The listing builds one solid part. Answer for the finished solid, in the listing's coordinates (mm). Face numbers are marked on the shaded views. A direction names the side the tool comes from. Give positions to 0.01 mm unless a question says otherwise; leave off trailing zeros. Write each loop counter-clockwise with the first axis right and the second up, starting at its lowest first coordinate (ties: lowest second). Pieces come first, ordered by that corner, then holes. Notation, with made-up numbers: (31, 26) - (74, 26) arc R20 ccw to (74, 32) - close; hole circle Ø4 at (51.5, -29.5). An arc over 180 degrees is marked (long way). Use a Markdown table: item, result. Add a question column.
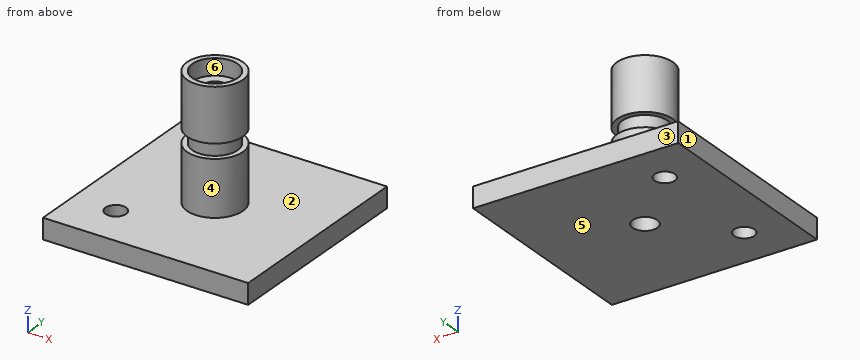
Autodesk Inventor part; units mm, degrees
ref_plane "Plano de trabajo1" through (0, 0, 13.5) normal (0, 0, -1) x (-1, 0, 0)
ref_plane "YZ Plane" through (0, 0, 0) normal (1, 0, 0) x (0, 1, 0)
ref_plane "XZ Plane" through (0, 0, 0) normal (0, 1, 0) x (-1, 0, 0)
sketch "Boceto1" plane through (0, 0, 0) normal (0, 0, 1) x (1, 0, 0)
  circle A0 centre (0, 0) radius 6.8
  dimension "d0" = 13.6
extrude "Extrusión1" add sketch "Boceto1" along normal blind 30
ref_plane "Plano de trabajo1" through (0, 0, 13.5) normal (0, 0, -1) x (-1, 0, 0)
sketch "Boceto2" plane through (0, 0, 13.5) normal (0, 0, -1) x (-1, 0, 0)
  circle A0 centre (0, 0) radius 5.5
  circle A1 centre (0, 0) radius 7
  dimension "d4" = 11
  dimension "d5" = 14
extrude "Extrusión2" cut sketch "Boceto2" against normal blind 3.5
sketch "Boceto3" plane through (0, 0, 0) normal (0, 0, -1) x (-1, 0, 0)
  line L0 (-25, 25) -> (25, 25)
  line L1 (25, 25) -> (25, -25)
  line L2 (25, -25) -> (-25, -25)
  line L3 (-25, -25) -> (-25, 25)
  line L4 (-25, 25) -> (25, -25) construction
  line L5 (25, 25) -> (-25, -25) construction
  line L6 (25, 25) -> (15, 25)
  line L7 (15, 25) -> (15, 16.75)
  line L8 (16.95, 14.8) -> (25, 14.8)
  line L9 (25, 14.8) -> (25, 25)
  line L10 (25, -25) -> (15, -25)
  line L11 (15, -25) -> (15, -16.75)
  line L12 (16.95, -14.8) -> (25, -14.8)
  line L13 (25, -14.8) -> (25, -25)
  line L14 (-25, 25) -> (-14.8, 25)
  line L15 (-14.8, 25) -> (-14.8, 16.95)
  line L16 (-16.75, 15) -> (-25, 15)
  line L17 (-25, 15) -> (-25, 25)
  line L18 (-25, -25) -> (-15, -25)
  line L19 (-15, -25) -> (-15, -16.9397)
  line L20 (-16.75, -15) -> (-25, -15)
  line L21 (-25, -15) -> (-25, -25)
  circle A0 centre (14.5004, 14.3004) radius 2.5
  circle A1 centre (14.5004, -14.3004) radius 2.5
  circle A2 centre (-14.8, 15) radius 1.95
  circle A3 centre (-14.8, -15) radius 1.95
  point P0 (0, 0)
  dimension "d8" = 50
  dimension "d9" = 50
  dimension "d18" = 5
  dimension "d19" = 5
  dimension "d20" = 3.9
  dimension "d21" = 3.9
  dimension "d24" = 8.25
  dimension "d25" = 8.05
  dimension "d26" = 8.25
  dimension "d27" = 8.0603
  dimension "d28" = 8.25
  dimension "d29" = 8.05
  dimension "d30" = 8.25
  dimension "d31" = 8.05
extrude "Extrusión3" add sketch "Boceto3" along normal blind 5 contours L0 L15 A2 L16 L3 | L0 L7 A0 L8 L1 L12 A1 L11 L2 L19 A3 L20 L3 L16 A2 L15 | L0 L1 L8 A0 L7 | L20 A3 L19 L2 L3 | L1 L2 L11 A1 L12
sketch "Boceto4" plane through (0, 0, 13.5) normal (0, 0, -1) x (-1, 0, 0)
  point P0 (0, 0)
sketch "Boceto5" plane through (0, 0, -5) normal (0, 0, -1) x (-1, 0, 0)
  circle A0 centre (0, 0) radius 5.5
  circle A1 centre (0, 0) radius 3
  dimension "d32" = 6
extrude "Extrusión4" cut sketch "Boceto5" against normal blind 33 contours A1
sketch "Boceto6" plane through (0, 0, 30) normal (0, 0, 1) x (1, 0, 0)
  circle A0 centre (0, 0) radius 5.5
  dimension "d35" = 11
extrude "Extrusión5" cut sketch "Boceto6" against normal blind 4
sketch "Boceto7" plane through (0, 0, -5) normal (0, 0, -1) x (-1, 0, 0)
  circle A0 centre (-14.8, -15) radius 1.95
  circle A1 centre (-14.8, 15) radius 1.95
  point P0 (0, 0)
extrude "Extrusión6" add sketch "Boceto7" against normal up to surface (5 mm away)
properties part number "pieza_2_vinculacion"
1. The part is cut by section D-D (y = 19.5). Give the vertices of the cut face in (x, z).
2. Given P1, Ø4, axis at x = 9, y = -17, coming from the +Z side, flat-ended and moving along its own axis, determine where the tip first touches the part or whether it passes through.
3. The part is cut by section C-C (z = 18.5). Give the vertices of the cut face in (x, y).
4. Consider L1, parallel to Y at x = 0, z = 11; L2, parallel to Z at x = -5.5, y = 3; L3, parallel to Y at x = 0, z = 29. Determine where each line is inside the solid, lowest interval first. Write a range as [from, to].
5. For a pull along Y with two mould halves and no side action, classify the marked faces 3, 4, 5 and 6 as released by +Y, released by -Y, zero draft, split by the parting line, or undercut.
6. Which of the six approach directions +Z, -Z, +X, -X, +Y, -Y give full straight-line access (tool end or side, diameter ignored) to the marked faces 1 and 2?
7. The part is cut by section A-A (x = 0). Give the vertices of the cut face in (y, z), and give its area (3 significant figures).
Check values:
| question | item | result |
|---|---|---|
| 1 | outline | (-25, -5) - (25, -5) - (25, 0) - (-25, 0) - close |
| 2 | P1 | stops at z = 0 |
| 3 | outline | circle Ø13.6 at (0, 0); hole circle Ø6 at (0, 0) |
| 4 | L1 | y = [-6.8, -3], [3, 6.8] |
| 4 | L2 | z = [-5, 13.5], [17, 30] |
| 4 | L3 | y = [-6.8, -5.5], [5.5, 6.8] |
| 5 | face 3 | released by +Y |
| 5 | face 4 | split by the parting line |
| 5 | face 5 | zero draft |
| 5 | face 6 | undercut |
| 6 | face 1 | +Z, -Z, -X, +Y, -Y |
| 6 | face 2 | +Z |
| 7 | outline | (-25, -5) - (-3, -5) - (-3, 26) - (-5.5, 26) - (-5.5, 30) - (-6.8, 30) - (-6.8, 17) - (-5.5, 17) - (-5.5, 13.5) - (-6.8, 13.5) - (-6.8, 0) - (-25, 0) - close; (3, -5) - (25, -5) - (25, 0) - (6.8, 0) - (6.8, 13.5) - (5.5, 13.5) - (5.5, 17) - (6.8, 17) - (6.8, 30) - (5.5, 30) - (5.5, 26) - (3, 26) - close |
| 7 | area | 419 mm2 |
